The listing builds one solid part. Answer for the finished solid, in the listing's coordinates (mm). A direction names the side the tool comes from. Give positions to 0.01 mm unless a question says otherwise; leave off trailing zeros. Order: outer loops, then holes, each group sorted by start corner. A loop starts at its lowest first (then second) coordinate and runs counter-clockwise, first axis right, second up. Notation, with made-up numbers: (77.25, -3) - (104.25, -3) arc R22 ccw to (104.25, 15) - close; hole circle Ø1 at (8.25, 63.5). An arc over 180 degrees is marked (long way). Use a Markdown table: item, result. Add a question column.
1) Find section A-A, the plane z = 0. Determine the outline of the cut face in (x, y).
2) For faces 1 (the face through (1, 1, 10)), 2 (the face through (18, 1, 7.5)), 3 (the face through (-15, 1, 0)), determine the directions among +Z, -Z, +X, -X, +Y, -Y from which every point of the face is accessible in a straight line to the end or side of a thin tool.
3) The mould has two halves that part along X. Classify faces 4 (the face through (-19.643, 1.232, -12.9)), 5 (the face through (24.393, 1.268, 9.193)), 6 (the face through (6, 1, 0)): released by +X, released by -X, zero draft, split by the parting line, or undercut.
4) Find section B-B, the plane x = -8.5. Determine the outline of the cut face in (y, z).
5) Find section C-C, the plane x = 18. Determine the outline of the cut face in (y, z).
6) Straight lines are drawn through the part: line 1 (X direction, y = 0.95, z = 0); line 2 (Z direction, x = 5.5, y = 0.7); line 3 (Z direction, x = 3, y = 0.3). For each, find the intervals that lie inside material, in ascending order.
7) Flat-ended cylindrical pins translate along their axes: pin 1 (0.8 mm diameter, centred on y = 1.5, z = 9, fed in from -X); pin 2 (1 mm diameter, centred on y = 0.5, z = 3.5, fed in from +X); pin 3 (0.8 mm diameter, centred on y = 1, z = 8.5, fed in from +X); pin 4 (9.5 mm diameter, centred on x = 0, z = 0, fed in from -Y). Find the tip coordinate at first contact, or state that the pin passes through.
Autodesk Inventor part; units mm, degrees
ref_plane "YZ Plane" through (0, 0, 0) normal (1, 0, 0) x (0, 1, 0)
ref_plane "XZ Plane" through (0, 0, 0) normal (0, 1, 0) x (-1, 0, 0)
ref_plane "XY Plane" through (0, 0, 0) normal (0, 0, 1) x (1, 0, 0)
sketch "スケッチ1" plane through (0, 0, 0) normal (0, 1, 0) x (-1, 0, 0)
  circle A0 centre (0, 0) radius 6
  line L0 (0, 3) -> (15, 3)
  line L1 (15, 3) -> (15, -3)
  line L2 (15, -3) -> (0, -3)
  line L3 (0, -3) -> (0, 3) construction
  line L4 (23.5, 10) -> (-25.7338, 10)
  line L5 (-25.7338, 10) -> (-25.7338, -10) construction
  line L6 (-25.7338, -10) -> (23.5, -10)
  line L7 (23.5, -10) -> (23.5, 10) construction
  circle A1 centre (0, 0) radius 23.5
  circle A2 centre (-47, 0) radius 23.5
  line L8 (-23.5, 10) -> (-23.5, 0)
  line L9 (0, -23.5) -> (-47, -23.5)
  line L10 (0, 23.5) -> (-47, 23.5)
  point P0 (-25.7338, 0)
  point P1 (20.3516, -11.75)
  point P2 (-26.6484, -11.75)
  point P3 (5.1962, -3)
  point P4 (5.1962, 3)
  point P5 (21.2662, 10)
  point P6 (-21.2662, 10)
  dimension "d0" = 12
  dimension "d1" = 15
  dimension "d2" = 6
  dimension "d3" = 20
  dimension "d4" = 47
  dimension "d5" = 47
  dimension "d6" = 47
extrude "押し出し1" add sketch "スケッチ1" along normal blind 2.5 contours L8 A2 L4 | L4 A1 L8 | L4 A1 L6 | A1 L6 A2 | A1 L9 A2 L6 | L6 A1
fillet "フィレット2" radius 2 3 edges at (47, 1.25, -23.5) (25.7338, 1.25, 10) (-21.2662, 1.25, 10)
sketch "スケッチ2" plane through (0, 2.5, 0) normal (0, 1, 0) x (1, 0, 0)
  line L0 (-19.9562, -10) -> (22.7874, -10)
  line L1 (-19.9562, -10) -> (22.7874, -10)
  line L2 (22.7874, -10) -> (22.7874, -7.5)
  line L3 (22.7874, -7.5) -> (-19.9562, -7.5)
  line L4 (-19.9562, -7.5) -> (-19.9562, -10)
  line L5 (-19.9562, -10) -> (-9.9562, -10)
  line L6 (-9.9562, -10) -> (-9.9562, -7.5)
  line L7 (-9.9562, -7.5) -> (-19.9562, -7.5)
  line L8 (-19.9562, -7.5) -> (-19.9562, -10)
  line L9 (22.7874, -10) -> (12.7874, -10)
  line L10 (12.7874, -10) -> (12.7874, -7.5)
  line L11 (12.7874, -7.5) -> (22.7874, -7.5)
  line L12 (22.7874, -7.5) -> (22.7874, -10)
  point P0 (0, 0)
  dimension "d13" = 2.5
  dimension "d14" = 10
  dimension "d15" = 10
extrude "押し出し2" cut sketch "スケッチ2" against normal through all contours L4 L3 L6 L0 | L10 L3 L2 L0
properties part number "皿"
The answers:
| question | item | result |
|---|---|---|
| 1 | outline | (-23.5, 0) - (-15, 0) - (-15, 2.5) - (-23.5, 2.5) - close; (6, 0) - (23.5, 0) - (23.5, 2.5) - (6, 2.5) - close |
| 2 | face 1 | +Z, +X, -X, +Y, -Y |
| 2 | face 2 | +Z, +Y, -Y |
| 2 | face 3 | +Y, -Y |
| 3 | face 4 | released by -X |
| 3 | face 5 | released by +X |
| 3 | face 6 | undercut |
| 4 | outline | (0, -21.91) - (2.5, -21.91) - (2.5, -3) - (0, -3) - close; (0, 3) - (2.5, 3) - (2.5, 10) - (0, 10) - close |
| 5 | outline | (0, -23.5) - (2.5, -23.5) - (2.5, 7.5) - (0, 7.5) - close |
| 6 | line 1 | -23.5 to -15, 6 to 23.5 |
| 6 | line 2 | -23.5 to -2.4, 2.4 to 10 |
| 6 | line 3 | -23.5 to -5.2, 5.2 to 10 |
| 7 | pin 1 | x = -21.87 |
| 7 | pin 2 | x = 23.84 |
| 7 | pin 3 | x = 24.78 |
| 7 | pin 4 | through |
